```python
from build123d import *

# Parameters (mm, degrees)
SKETCH_W        = 47
SKETCH_H        = 90
PAD_DEPTH       = 35.75
THICKNESS_T     = 4
SKETCH001_R     = 0.025
POCKET_DEPTH    = 5
SKETCH002_W     = 7
SKETCH002_H     = 42
POCKET001_DEPTH = 5
SKETCH003_W     = 5.5
SKETCH003_H     = 60
PAD001_DEPTH    = 7
PAD001_FACE4_W  = 90
PAD001_FACE4_H  = 47
POCKET002_DEPTH = 4
SKETCH004_W     = 31
SKETCH004_H     = 40
POCKET003_DEPTH = 11.3
SKETCH005_W     = 90
SKETCH005_H     = 5
PAD002_DEPTH    = 32
PAD003_DEPTH    = 20
POCKET004_DEPTH = 7


with BuildPart() as part:
    # Sketch → Pad (new body)
    with BuildSketch(Plane.XY):
        with Locations((23.5, 45)):
            Rectangle(SKETCH_W, SKETCH_H)
    extrude(amount=PAD_DEPTH)

    # Thickness
    thickness_openings = [part.faces().sort_by_distance(p)[0] for p in [
        (23.5, 45, 0),
    ]]
    offset(amount=THICKNESS_T, openings=thickness_openings)

    # Sketch001 (on Face10 of Thickness) → Pocket (cut)
    with BuildSketch(Plane.YZ.offset(51)):
        with Locations((27, 19)):
            Circle(SKETCH001_R)
    extrude(amount=-POCKET_DEPTH, mode=Mode.SUBTRACT)

    # Sketch002 (on Face24 of Pocket) → Pocket001 (cut)
    with BuildSketch(Plane.XY.offset(39.75)):
        with Locations((27.5, 68)):
            Rectangle(SKETCH002_W, SKETCH002_H)
    extrude(amount=-POCKET001_DEPTH, mode=Mode.SUBTRACT)

    # Sketch003 (on Face28 of Pocket001) → Pad001 (join)
    with BuildSketch(Plane.XY.offset(39.75)):
        with Locations((18.05, 59)):
            Rectangle(SKETCH003_W, SKETCH003_H)
        with Locations((36.95, 59)):
            Rectangle(SKETCH003_W, SKETCH003_H)
    extrude(amount=PAD001_DEPTH)

    # Pad001 Face4 → Pocket002 (cut)
    with BuildSketch(Plane(origin=(23.5, 45, 0), x_dir=(0, -1, 0), z_dir=(0, 0, -1))):
        with BuildLine():
            ThreePointArc((-45, 27.5), (-47.828427, 26.328427), (-49, 23.5))
            Line((-49, 23.5), (-49, -23.5))
            ThreePointArc((-49, -23.5), (-47.828427, -26.328427), (-45, -27.5))
            Line((-45, -27.5), (45, -27.5))
            ThreePointArc((45, -27.5), (47.828427, -26.328427), (49, -23.5))
            Line((49, -23.5), (49, 23.5))
            ThreePointArc((49, 23.5), (47.828427, 26.328427), (45, 27.5))
            Line((45, 27.5), (-45, 27.5))
        make_face()
        Rectangle(PAD001_FACE4_W, PAD001_FACE4_H, mode=Mode.SUBTRACT)
    extrude(amount=-POCKET002_DEPTH, mode=Mode.SUBTRACT)

    # Sketch004 (on Face12 of Pocket002) → Pocket003 (cut)
    with BuildSketch(Plane.YZ.offset(51)):
        with Locations((72.5, 24)):
            Rectangle(SKETCH004_W, SKETCH004_H)
    extrude(amount=-POCKET003_DEPTH, mode=Mode.SUBTRACT)

    # Sketch005 (on Face11 of Pocket003) → Pad002 (join)
    with BuildSketch(Plane(origin=(-4, 0, 0), x_dir=(0, -1, 0), z_dir=(-1, 0, 0))):
        with Locations((-45, 6.5)):
            Rectangle(SKETCH005_W, SKETCH005_H)
    extrude(amount=PAD002_DEPTH)

    # Sketch006 (on Face47 of Pad002) → Pad003 (join)
    with BuildSketch(Plane.XZ.offset(-29)):
        Polygon((15.3, 50.25), (34.2, 50.25), (39.7, 50.25), (39.7, 46.75), (34.2, 46.75), (34.2, 43.15), (15.3, 43.15), align=None)
    extrude(amount=-PAD003_DEPTH)

    # Sketch007 (on Face49 of Pad003) → Pocket004 (cut)
    with BuildSketch(Plane.XY.offset(46.75)):
        Polygon((20.8, 89), (18.8, 89), (20.8, 49), align=None)
        Polygon((34.2, 89), (36.2, 89), (34.2, 49), align=None)
    extrude(amount=-POCKET004_DEPTH, mode=Mode.SUBTRACT)


solid = part.part
```
Work out the finished part from the listing and answer in its coordinate system (mm). A direction names the side the tool comes from. Give positions to 0.01 mm unless a question says otherwise; leave off trailing zeros. Order: outer loops, then holes, each group sorted by start corner. A loop starts at its lowest first (then second) coordinate and runs counter-clockwise, first axis right, second up. Notation, with made-up numbers: (32.5, 74) -> (61.5, 74) arc R20 cw to (61.5, 87) -> close; hole circle Ø3 at (-22, 74.5). An arc over 180 degrees is marked (long way). Answer as CSV lines item,"result". Start each with the question number.
(1) Which of the six approach directions +Z, -Z, +X, -X, +Y, -Y give full straight-line access (tool end or side, diameter ignored) to faces 4 (the flat face through (27, 89, 38)), 5 (the flat face through (-20, 90, 6)), 6 (the flat face through (-4, 44, 22))?
(2) Each of these flat-tipped pins is pushed along its axis until it touches: pin 1 Ø6 at (x, y) = (37, 66) entering from +Z; pin 2 Ø2 at (x, z) = (26.5, 37) entering from -Y; pin 3 Ø1.7 at (y, z) = (42.5, 42) entering from -X. Where does it stop, or does it pass through?
(3) Section C-C, the plane z = 41 is taken. Write down the section's boundary in (x, y).
(4) Section B-B, the plane y = 85 is taken. Write down the section's boundary in (x, z), plus the area to 3 significant figures.
(5) Section A-A, the plane x = 26.5 is taken. Write down the section's boundary in (y, z), plus the area to 3 significant figures.
(6) Section D-D, the plane x = 44 is taken. Write down the section's boundary in (y, z).
(7) For a pull along X with two mould halves and no side action, classify faces 1 (the flat face through (23, 90, 20)), 2 (the cylindrical face through (49.859, 28.899, 38.547)), 3 (the cylindrical face through (-2.859, 92.797, 20.097)) as released by +X, released by -X, zero draft, split by the parting line, or undercut.
(8) Consider line 1 along X through (y, z) = (40, 6.5); line 2 along Y through (x, z) = (8, 17); line 3 along X through (y, z) = (11.5, 22.5). Determine where each line is inside the solid, lowest interval first.
Entries:
1,face 4,"+Z, -Z"
1,face 5,"+Z, -Z, -X, +Y"
1,face 6,"+Z, -X, +Y, -Y"
2,pin 1,"z = 46.75"
2,pin 2,"y = -3.99"
2,pin 3,"x = 15.3"
3,outline,"(15.3, 29) -> (20.8, 29) -> (20.8, 49) -> (18.8, 89) -> (15.3, 89) -> close; (34.2, 29) -> (39.7, 29) -> (39.7, 89) -> (36.2, 89) -> (34.2, 49) -> close"
4,outline,"(-36, 4) -> (0, 4) -> (0, 35.75) -> (24, 35.75) -> (24, 39.75) -> (19, 39.75) -> (19, 46.75) -> (15.3, 46.75) -> (15.3, 39.75) -> (0, 39.75) arc R4 ccw to (-4, 35.75) -> (-4, 9) -> (-36, 9) -> close; (31, 35.75) -> (39.7, 35.75) -> (39.7, 46.75) -> (36, 46.75) -> (36, 39.75) -> (31, 39.75) -> close"
4,area,"482 mm²"
5,outline,"(-4, 4) -> (0, 4) -> (0, 35.75) -> (47, 35.75) -> (47, 39.75) -> (0, 39.75) arc R4 ccw to (-4, 35.75) -> close; (29, 43.15) -> (49, 43.15) -> (49, 50.25) -> (29, 50.25) -> close; (89, 35.75) -> (90, 35.75) -> (90, 4) -> (94, 4) -> (94, 35.75) arc R4 ccw to (90, 39.75) -> (89, 39.75) -> close"
5,area,"613 mm²"
6,outline,"(-4, 4) -> (0, 4) -> (0, 35.75) -> (57, 35.75) -> (57, 39.75) -> (0, 39.75) arc R4 ccw to (-4, 35.75) -> close; (88, 35.75) -> (90, 35.75) -> (90, 4) -> (94, 4) -> (94, 35.75) arc R4 ccw to (90, 39.75) -> (88, 39.75) -> close"
7,face 1,"undercut"
7,face 2,"released by +X"
7,face 3,"released by -X"
8,line 1,"-36 to 0, 47 to 51"
8,line 2,"-4 to 0, 90 to 94"
8,line 3,"-4 to 0, 47 to 51"
